The figure shows three views and two pictorial views of one solid part (mm, origin at its lowest corner). Answer the questions. Round coordinates to 2 decimals unless told otherwise and drop trailing zeros. Order: outer loops, then holes, each group sorted by start corner. A loop starts at its lowest first (then second) coordinate and runs counter-clockwise, first axis right, second up.
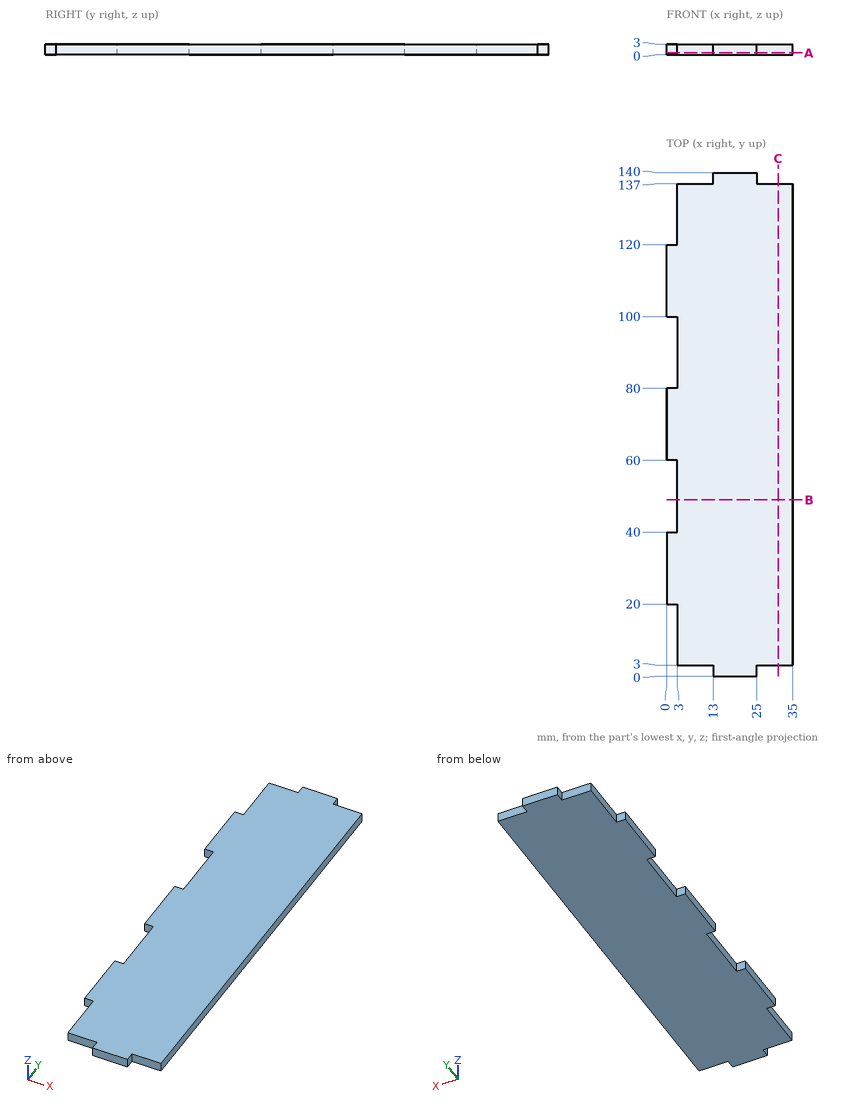
Item 1: Find the intervals of material crossed by line 1 along X through (y, z) = (15, 2.8); line 2 along Y through (x, z) = (30, 0.8), in increasing order.
Item 2: Find section B-B (y = 49). Write down the section's boundary in (x, z).
Item 3: Given pin 1 (1 mm diameter, centred on y = 54, z = 2, fed in from -X); pin 2 (1.5 mm diameter, centred on x = 2, z = 2, fed in from +Y); pin 3 (0.9 mm diameter, centred on x = 30.5, z = 1, fed in from -Y), each flat-ended and moving along its own axis, determine where each tip first touches the part or whether it passes through.
Item 4: Find section C-C (x = 31). Write down the section's boundary in (y, z), plus the area to 3 significant figures.
Item 5: Find section A-A (z = 0.55). Write down the section's boundary in (x, y).
Model answer:
1. line 1: x = 3 to 35
1. line 2: y = 3 to 137
2. outline: (3, 0) - (35, 0) - (35, 3) - (3, 3) - close
3. pin 1: stops at x = 3
3. pin 2: stops at y = 120
3. pin 3: stops at y = 3
4. outline: (3, 0) - (137, 0) - (137, 3) - (3, 3) - close
4. area: 402 mm2
5. outline: (0, 20) - (3, 20) - (3, 3) - (13, 3) - (13, 0) - (25, 0) - (25, 3) - (35, 3) - (35, 137) - (25, 137) - (25, 140) - (13, 140) - (13, 137) - (3, 137) - (3, 120) - (0, 120) - (0, 100) - (3, 100) - (3, 80) - (0, 80) - (0, 60) - (3, 60) - (3, 40) - (0, 40) - close
